```python
from build123d import *

# Parameters (mm, degrees)
SKETCH1_R           = 3
BOSS_EXTRUDE1_DEPTH = 2
SKETCH2_R           = 2.5
BOSS_EXTRUDE2_DEPTH = 2
SKETCH3_R           = 3.5
BOSS_EXTRUDE3_DEPTH = 4
SKETCH4_R           = 5
BOSS_EXTRUDE4_DEPTH = 4
BOSS_EXTRUDE4_TAPER = 20


with BuildPart() as part:
    # Sketch1 → Boss-Extrude1 (new body)
    with BuildSketch(Plane(origin=(0, 0, 0), x_dir=(1, 0, 0), z_dir=(0, 1, 0))):
        Circle(SKETCH1_R)
    extrude(amount=BOSS_EXTRUDE1_DEPTH)

    # Sketch2 → Boss-Extrude2 (add)
    with BuildSketch(Plane.XZ):
        Circle(SKETCH2_R)
    extrude(amount=BOSS_EXTRUDE2_DEPTH)

    # Sketch3 → Boss-Extrude3 (add)
    with BuildSketch(Plane.XZ.offset(2)):
        Circle(SKETCH3_R)
    extrude(amount=BOSS_EXTRUDE3_DEPTH)

    # Sketch4 → Boss-Extrude4 (add)
    with BuildSketch(Plane.XZ.offset(6)):
        Circle(SKETCH4_R)
    extrude(amount=BOSS_EXTRUDE4_DEPTH, taper=BOSS_EXTRUDE4_TAPER)


solid = part.part
```
Design review of the part built by this model. Coordinates are the model's own, in mm. A direction names the side the tool comes from. Give positions to 0.01 mm unless a question says otherwise; leave off trailing zeros. Loops run counter-clockwise (first coordinate to the right, second up) from the corner with the lowest first, then second, coordinate; pieces in that order, holes last. Notation, with made-up numbers: (78, 73.25) -> (97, 73.25) arc R14 cw to (97, 94.25) -> close; hole circle Ø9 at (8.5, -26). An arc over 180 degrees is marked (long way). One line per item, written item: value.
Q1. Machinability: for faces 1 (the cylindrical face through (-0.54, -0.99, -2.44)), 2 (the flat face through (0, 2, 0)), 3 (the cylindrical face through (-3, 1, 0)), which of the approach directions +Z, -Z, +X, -X, +Y, -Y give a long, thin tool a straight path to every point of the face, cutting with its end or side? Answer none if there is none.
Numbers:
face 1: none
face 2: +Z, -Z, +X, -X, +Y
face 3: +Y
Q2. We need section C-C on y = 0.5. Give the boundary of the cut face in (x, z), and give its area (3 significant figures).
Numbers:
outline: circle Ø6 at (0, 0)
area: 28.3 mm^2
Q3. For L1, parallel to Z at x = 0, y = -0.75; L2, parallel to Y at x = 2, z = -1.75; L3, parallel to Y at x = -2.75, z = -2, list the stretches that pass through material, from the lowest coordinate up.
Numbers:
L1: z = -2.5 to 2.5
L2: y = -10 to -2, 0 to 2
L3: y = -10 to -2
Q4. We need section A-A on x = 0. Give the boundary of the cut face in (y, z), and give its area (3 significant figures).
Numbers:
outline: (-10, -3.54) -> (-6, -5) -> (-6, -3.5) -> (-2, -3.5) -> (-2, -2.5) -> (0, -2.5) -> (0, -3) -> (2, -3) -> (2, 3) -> (0, 3) -> (0, 2.5) -> (-2, 2.5) -> (-2, 3.5) -> (-6, 3.5) -> (-6, 5) -> (-10, 3.54) -> close
area: 84.2 mm^2
Q5. We need section B-B on y = -4.75. Give the boundary of the cut face in (x, z).
Numbers:
outline: circle Ø7 at (0, 0)
Q6. For pin 1 Ø3 at (x, y) = (2.5, -3.5) entering from +Z; pin 2 Ø4 at (y, z) = (-2.5, 4) entering from +X; pin 3 Ø2 at (x, y) = (-3, -7.5) entering from +Z, all flat-tipped, find the tip position at first contact; note any pin that passes through.
Numbers:
pin 1: stops at z = 3.35
pin 2: stops at x = 2.87
pin 3: stops at z = 4.12
Q7. Draft analysis for pull direction Y (two halves, no side actions). For faces 4 (the flat face through (-2, 0, -2)), 5 (the flat face through (2.2, -6, -3.3)), 6 (the flat face through (2, -2, -2)), 7 (the flat face through (0, -10, 0)), state which applies: pulls with the +Y half, pulls with the -Y half, needs draft (parallel to the pull), parting line crosses it, or undercut.
Numbers:
face 4: undercut
face 5: pulls with the +Y half
face 6: undercut
face 7: pulls with the -Y half
